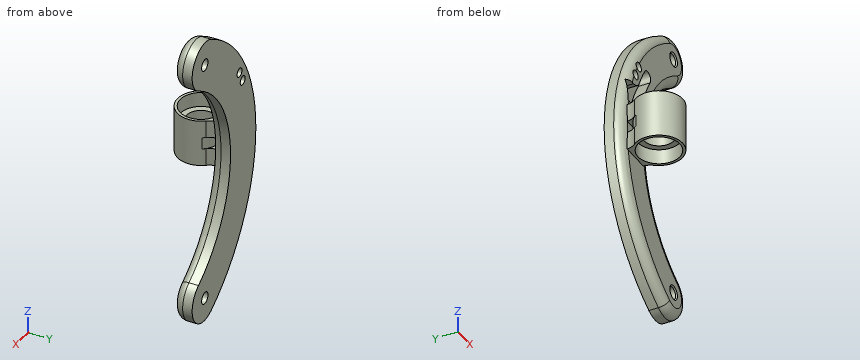
from build123d import *

# Parameters (mm, degrees)
SENSORARMATURE_DEPTH                  = 12.7
SENSORARMATURE_DEPTH_BACK             = 12.7
SKETCH2_R                             = 7.9375
SKETCH2_R_2                           = 4
SKETCH2_R_3                           = 2.38125
SKETCH15_R                            = 11.25
BEARINGRACE1_DEPTH                    = 8
SKETCH16_R                            = 11.25
BEARINGRACE2_DEPTH                    = 8
CUT_EXTRUDE3_DEPTH                    = 188.895496905
FILLET1_R                             = 9.525
MAINSENSORINSET_DEPTH                 = 6.35
F_10_0_1935_DIAMETER_HOLE1_D          = 4.9149
F_1_4_0_25_DIAMETER_HOLE1_D           = 6.35
F_1_4_0_25_DIAMETER_HOLE1_CSINK_D     = 7.62
F_1_4_0_25_DIAMETER_HOLE1_CSINK_ANGLE = 90
CUT_EXTRUDE6_DEPTH                    = 132.65094541
CUT_EXTRUDE6_DEPTH_BACK               = 132.65094541
FILLET2_ANGLE                         = 180
FILLET2_2_ANGLE                       = 180


with BuildPart() as part:
    # Sketch1 → MainAttachmentRing (revolve)
    with BuildSketch(Plane.XY, mode=Mode.PRIVATE) as mainattachmentring_sk:
        with BuildLine():
            Line((-64.29375, 0), (-64.29375, -5.08))
            ThreePointArc((-64.29375, -5.08), (-65.688653955, -8.447596045), (-69.05625, -9.8425))
            Line((-69.05625, -9.8425), (-84.93125, -9.8425))
            ThreePointArc((-84.93125, -9.8425), (-88.298846045, -8.447596045), (-89.69375, -5.08))
            Line((-89.69375, -5.08), (-89.69375, 0))
            Line((-89.69375, 0), (-64.29375, 0))
        make_face()
    revolve(mainattachmentring_sk.sketch.rotate(Axis((0, -6.614583333, 0), (0, 1, 0)), 270), axis=Axis((0, -6.614583333, 0), (0, 1, 0)))

    # Sketch2 → SensorArmature (add, two sides: drawn at the far end of the back side and taken through both)
    # profile 1 of 2: a face of its own
    with BuildSketch(Plane.XY.offset(-SENSORARMATURE_DEPTH_BACK)):
        with BuildLine():
            Line((-69.05625, -8.794346715), (-69.05625, -3.4925))
            Line((-69.05625, -3.4925), (-84.93125, -3.4925))
            Line((-84.93125, -3.4925), (-84.93125, -8.794346715))
            ThreePointArc((-84.93125, -8.794346715), (-85.455970986, -11.912134822), (-86.972321429, -14.686412409))
            ThreePointArc((-86.972321429, -14.686412409), (-76.99375, -35.2425), (-67.015178571, -14.686412409))
            ThreePointArc((-67.015178571, -14.686412409), (-68.531529014, -11.912134822), (-69.05625, -8.794346715))
        make_face()
        with Locations((-76.99375, -22.5425)):
            Circle(SKETCH2_R, mode=Mode.SUBTRACT)
    # profile 2 of 2: a face of its own
    with BuildSketch(Plane.XY.offset(-SENSORARMATURE_DEPTH_BACK)):
        with Locations((-76.99375, -22.5425)):
            Circle(SKETCH2_R_2)
        with Locations((-76.99375, -22.5425)):
            Circle(SKETCH2_R_3, mode=Mode.SUBTRACT)
    extrude(amount=SENSORARMATURE_DEPTH + SENSORARMATURE_DEPTH_BACK)


with BuildPart() as sensorarmature_kept_piece:
    # of the separate pieces the step leaves, the one the design keeps (sensorarmature_pieces_kept)
    add(part.part.solids().sort_by_distance((0, 0, -64.29375))[0])

    # Sketch15 → BearingRace1 (cut)
    with BuildSketch(Plane.XY.offset(12.7)):
        with Locations((-76.99375, -22.5425)):
            Circle(SKETCH15_R)
    extrude(amount=-BEARINGRACE1_DEPTH, mode=Mode.SUBTRACT)

    # Sketch16 → BearingRace2 (cut)
    with BuildSketch(Plane(origin=(0, 0, -12.7), x_dir=(-1, 0, 0), z_dir=(0, 0, -1))):
        with Locations(Location((76.99375, -22.5425, 0), (0, 0, 180))):
            Circle(SKETCH16_R)
    extrude(amount=-BEARINGRACE2_DEPTH, mode=Mode.SUBTRACT)

    # Sketch17 → Cut-Extrude3 (cut, through all)
    with BuildSketch(Plane(origin=(65.0875, 22.225, 0), x_dir=(0, 0, 1), z_dir=(-1, 0, 0))):
        with BuildLine():
            Line((2.825941823, -32.0675), (3.175, -32.0675))
            Line((3.175, -32.0675), (3.175, -33.655))
            Line((3.175, -33.655), (-3.175, -33.655))
            Line((-3.175, -33.655), (-3.175, -32.0675))
            Line((-3.175, -32.0675), (-2.825941823, -32.0675))
            add(Edge.make_bspline(
                [(-2.825941823, -32.0675), (-0.941980608, -32.0675), (0.941980608, -32.0675), (2.825941823, -32.0675)],
                knots=[0, 0, 0, 0, 1, 1, 1, 1], degree=3))
        make_face()
    extrude(amount=CUT_EXTRUDE3_DEPTH, mode=Mode.SUBTRACT)

    # Fillet1
    # the kernel refuses this fillet: 9.525 mm, written as the material it takes off along each edge
    with BuildSketch(Plane(origin=(-68.684334549, -11.43, 3.175), x_dir=(-1, 0, 0), z_dir=(0, 0, -1))) as fillet1_piece_1:
        with BuildLine():
            CenterArc((5.559784794, -9.525), FILLET1_R, 90, 60)
            Line((-2.689107177, -4.7625), (-3.513996374, -4.28625))
            ThreePointArc((-3.513996374, -4.28625), (-2.417548835, -2.667205839), (-0.915308455, 0.263565329))
            Line((-0.915308455, 0.263565329), (0, 0.9525))
            Line((0, 0.9525), (5.559784794, 0.9525))
            Line((5.559784794, 0.9525), (5.559784794, 0))
        make_face()
    extrude(amount=6.35, mode=Mode.SUBTRACT)
    with BuildSketch(Plane(origin=(-85.303165451, -11.43, 3.175), x_dir=(1, 0, 0), z_dir=(0, 0, -1))) as fillet1_piece_2:
        with BuildLine():
            CenterArc((5.559784794, 9.525), FILLET1_R, 210, 60)
            Line((-2.689107177, 4.7625), (-3.513996374, 4.28625))
            ThreePointArc((-3.513996374, 4.28625), (-2.417548835, 2.667205839), (-0.915308455, -0.263565329))
            Line((-0.915308455, -0.263565329), (0, -0.9525))
            Line((0, -0.9525), (5.559784794, -0.9525))
            Line((5.559784794, -0.9525), (5.559784794, 0))
        make_face()
    extrude(amount=6.35, mode=Mode.SUBTRACT)

    # Sketch19 → MainSensorInset (cut)
    with BuildSketch(Plane.XZ.offset(9.8425)):
        with BuildLine():
            Line((-83.97634921, 15.875), (-68.998403727, 15.875))
            Line((-68.998403727, 15.875), (-68.998403727, 23.64608578))
            ThreePointArc((-68.998403727, 23.64608578), (-68.895293758, 24.785763339), (-68.589312408, 25.888429207))
            ThreePointArc((-68.589312408, 25.888429207), (-65.62931995, 32.672571163), (-62.000346171, 39.123670816))
            ThreePointArc((-62.000346171, 39.123670816), (-62.991085358, 43.50313264), (-67.370547181, 42.512393453))
            ThreePointArc((-67.370547181, 42.512393453), (-70.269181894, 37.52780703), (-72.79966532, 32.346606528))
            ThreePointArc((-72.79966532, 32.346606528), (-75.142159242, 29.600748947), (-78.602628968, 28.575))
            Line((-78.602628968, 28.575), (-83.97634921, 28.575))
            Line((-83.97634921, 28.575), (-83.97634921, 15.875))
        make_face()
    extrude(amount=-MAINSENSORINSET_DEPTH, mode=Mode.SUBTRACT)

    # #10 (0.1935) Diameter Hole1 (through all)
    with Locations(Plane(origin=(0, -9.8425, 0), x_dir=(-1, 0, 0), z_dir=(0, -1, 0))):
        with Locations((73.312376468, -41.275), (76.487376468, -34.925)):
            Hole(F_10_0_1935_DIAMETER_HOLE1_D / 2)

    # 1/4 (0.25) Diameter Hole1 (through all)
    with Locations(Plane(origin=(0, -9.8425, 0), x_dir=(-1, 0, 0), z_dir=(0, -1, 0))):
        with Locations((-76.99375, 0), (38.496875, 66.678543433), (38.496875, -66.678543433), (0, 0)):
            CounterSinkHole(F_1_4_0_25_DIAMETER_HOLE1_D / 2, F_1_4_0_25_DIAMETER_HOLE1_CSINK_D / 2, counter_sink_angle=F_1_4_0_25_DIAMETER_HOLE1_CSINK_ANGLE)

    # Sketch28 → Cut-Extrude6 (cut, two sides: drawn at the far end of the back side and taken through both)
    with BuildSketch(Plane(origin=(0, 0, 0), x_dir=(1, 0, 0), z_dir=(0, 1, 0)).offset(-CUT_EXTRUDE6_DEPTH_BACK)):
        with BuildLine():
            Line((0, 0), (-32.146875, 55.680020805))
            ThreePointArc((-32.146875, 55.680020805), (-27.498352372, 73.028543433), (-44.846875, 77.677066061))
            Line((-44.846875, 77.677066061), (-52.641298624, 91.177403793))
            Line((-52.641298624, 91.177403793), (62.971207783, 117.188002958))
            Line((62.971207783, 117.188002958), (148.903396654, 11.630273141))
            Line((148.903396654, 11.630273141), (-6.989072656, -155.463930645))
            Line((-6.989072656, -155.463930645), (-55.413884825, -95.979663962))
            Line((-55.413884825, -95.979663962), (-44.846875, -77.677066061))
            ThreePointArc((-44.846875, -77.677066061), (-27.498352372, -73.028543433), (-32.146875, -55.680020805))
            Line((-32.146875, -55.680020805), (0, 0))
        make_face()
    extrude(amount=CUT_EXTRUDE6_DEPTH + CUT_EXTRUDE6_DEPTH_BACK, mode=Mode.SUBTRACT)

    # Fillet2: read off the stored shape, not the designer's step
    # Fillet2 outline → Fillet2 (revolve, cut)
    with BuildSketch(Plane(origin=(-38.496875, 0, 66.678543433), x_dir=(-0.4999999999999933, 0, 0.8660254037844425), z_dir=(-0.8660254037844425, 0, -0.4999999999999933))):
        with BuildLine():
            ThreePointArc((12.7, -5.08), (11.305096045, -8.447596045), (7.9375, -9.8425))
            Line((7.9375, -9.8425), (12.7, -9.8425))
            Line((12.7, -9.8425), (12.7, -5.08))
        make_face()
    revolve(axis=Axis((-38.496875, 0, 66.678543433), (0, 1, 0)), revolution_arc=FILLET2_ANGLE, mode=Mode.SUBTRACT)

    # Fillet2 2 outline → Fillet2 2 (revolve, cut)
    with BuildSketch(Plane(origin=(-38.496875, 0, -66.678543433), x_dir=(0.4999999999999988, 0, 0.8660254037844394), z_dir=(-0.8660254037844394, 0, 0.4999999999999988))):
        with BuildLine():
            ThreePointArc((12.7, -5.08), (11.305096045, -8.447596045), (7.9375, -9.8425))
            Line((7.9375, -9.8425), (12.7, -9.8425))
            Line((12.7, -9.8425), (12.7, -5.08))
        make_face()
    revolve(axis=Axis((-38.496875, 0, -66.678543433), (0, 1, 0)), revolution_arc=FILLET2_2_ANGLE, mode=Mode.SUBTRACT)


solid = sensorarmature_kept_piece.part
Verification items for the finished model (mm, model axes). Round coordinates to 2 decimals unless told otherwise and drop trailing zeros. Order: outer loops, then holes, each group sorted by start corner. A loop starts at its lowest first (then second) coordinate and runs counter-clockwise, first axis right, second up.
1. Go/stop test with flat-tipped pins: P1, Ø4, axis at y = -28, z = -3.5, coming from the +X side; P2, Ø11, axis at x = -68, z = 28.5, coming from the -Y side; P3, Ø4.5, axis at x = -81.5, y = -7, coming from the -Z side. Record where each tip stops, or that it passes through.
Final values:
P1: stops at x = -64.77
P2: stops at y = -9.84
P3: stops at z = -41.45
2. Thickness scan on L1, parallel to Z at x = -76, y = -32; L2, parallel to Z at x = -57.5, y = -6.5; L3, parallel to Y at x = -31, z = -64.5. Record the ranges inside material, lowest first.
Final values:
L1: z = -4.7 to 4.7
L2: z = -68.56 to -29.25, 29.25 to 68.56
L3: y = -9.84 to 0
3. Section check A-A on y = -29. Record the cut outline in (x, z).
Final values:
outline: (-87.93, -12.7) - (-86.21, -12.7) - (-86.21, -4.7) - (-81.61, -4.7) - (-81.61, 4.7) - (-86.21, 4.7) - (-86.21, 12.7) - (-87.93, 12.7) - close; (-72.38, -4.7) - (-67.78, -4.7) - (-67.78, -12.7) - (-66.06, -12.7) - (-66.06, 12.7) - (-67.78, 12.7) - (-67.78, 4.7) - (-72.38, 4.7) - close
4. Section check B-B on y = -18. Record the cut outline in (x, z).
Final values:
outline: (-88.85, -12.7) - (-87.29, -12.7) - (-87.29, -4.7) - (-83.5, -4.7) - (-83.5, 4.7) - (-87.29, 4.7) - (-87.29, 12.7) - (-88.85, 12.7) - close; (-70.48, -4.7) - (-66.7, -4.7) - (-66.7, -12.7) - (-65.13, -12.7) - (-65.13, 12.7) - (-66.7, 12.7) - (-66.7, 4.7) - (-70.48, 4.7) - close
